Could you check a few things on this model? Use its own coordinates, in mm. A direction names the side the tool comes from. Round coordinates to 2 decimals unless told otherwise and drop trailing zeros. Write each loop counter-clockwise with the first axis right and the second up, starting at its lowest first coordinate (ties: lowest second). Pieces come first, ordered by that corner, then holes. Notation, with made-up numbers: M -19.75,35.5 L 11.25,35.5 A13 cw 11.25,53.5 Z; hole C 20.25,-31 d5. An arc over 180 degrees is marked long. One line per question, with ' | ' between items. Start each with the question number.
```python
from build123d import *

# Parameters (mm, degrees)
SKETCH1_W           = 14.1
SKETCH1_H           = 14.1
BOSS_EXTRUDE1_DEPTH = 250.825
SKETCH2_W           = 10.1
SKETCH2_H           = 10.1
CUT_EXTRUDE1_DEPTH  = 255.432185656
SKETCH3_R           = 1.775
SKETCH3_R_2         = 2.358740524
CUT_EXTRUDE2_DEPTH  = 254.524349476
SKETCH4_R           = 1.775
CUT_EXTRUDE3_DEPTH  = 2
SKETCH5_R           = 1.775
CUT_EXTRUDE4_DEPTH  = 253.531071247


with BuildPart() as part:
    # Sketch1 → Boss-Extrude1 (new body)
    with BuildSketch(Plane.XY):
        with Locations((27.046996237, 18.639517713)):
            Rectangle(SKETCH1_W, SKETCH1_H)
    extrude(amount=BOSS_EXTRUDE1_DEPTH)

    # Sketch2 → Cut-Extrude1 (cut, through all)
    with BuildSketch(Plane.XY.offset(250.825)):
        with Locations((27.046996237, 18.639517713)):
            Rectangle(SKETCH2_W, SKETCH2_H)
    extrude(amount=-CUT_EXTRUDE1_DEPTH, mode=Mode.SUBTRACT)

    # Sketch3 → Cut-Extrude2 (cut, through all)
    with BuildSketch(Plane.XZ.offset(-11.589517713)):
        with Locations(Location((27.046996237, 237.825, 0), (0, 0, 270))):
            Circle(SKETCH3_R)
        with Locations(Location((27.046996237, 208.025, 0), (0, 0, 270))):
            Circle(SKETCH3_R)
        with Locations(Location((27.046996237, 8, 0), (0, 0, 270))):
            Circle(SKETCH3_R_2)
        with Locations(Location((27.046996237, 33, 0), (0, 0, 270))):
            Circle(SKETCH3_R_2)
    extrude(amount=-CUT_EXTRUDE2_DEPTH, mode=Mode.SUBTRACT)

    # Sketch4 → Cut-Extrude3 (cut)
    with BuildSketch(Plane.XZ.offset(-11.589517713)):
        with Locations(Location((27.046996237, 246.825, 0), (0, 0, 270))):
            Circle(SKETCH4_R)
    extrude(amount=-CUT_EXTRUDE3_DEPTH, mode=Mode.SUBTRACT)

    # Sketch5 → Cut-Extrude4 (cut, through all)
    with BuildSketch(Plane(origin=(34.096996237, 0, 0), x_dir=(0, 0, -1), z_dir=(1, 0, 0))):
        with Locations((-193.825, 18.639517713)):
            Circle(SKETCH5_R)
    extrude(amount=-CUT_EXTRUDE4_DEPTH, mode=Mode.SUBTRACT)


solid = part.part
```
1. Which directions (+Z, -Z, +X, -X, +Y, -Y) give clear straight access to the entire face, cutting with the end or side of a thin tool? Please do faces 1 (the face through (27, 25, 250.825)), 2 (the face through (27, 13.59, 127)).
2. If we mould it in two halves opening along Y, with no side actions, what happens to faces 3 (the face through (27, 11.59, 124)), 4 (the face through (27, 23.69, 127)), 5 (the face through (34.097, 19, 124))? For each: released by +Y, released by -Y, zero draft, split by the parting line, or undercut.
3. I need wall thicknesses on line 1 along X through (y, z) = (14, 139.5); line 2 along Y through (x, z) = (25.75, 39); line 3 along X through (y, z) = (13.1, 8). Which ranges of each line are inside material? Lowest first, please. Write a range as from..to.
4. Suppose I cut it at A-A (z = 8). Write out the boundary of the cut face in (x, y).
5. Suppose I cut it at B-B (z = 131). Write out the boundary of the cut face in (x, y), and give its area (3 significant figures).
6. I'm going to push flat-ended pins straight in: P1, Ø2, axis at x = 27.5, y = 14.5, coming from the -Z side; P2, Ø4, axis at x = 25.5, y = 20, coming from the +Z side. Where does each tip first touch, or does it pass through?
Computed:
1) face 1: +Z, +X, -X, +Y, -Y | face 2: +Z, -Z
2) face 3: released by -Y | face 4: undercut | face 5: zero draft
3) line 1: x = 20..22, 32.1..34.1 | line 2: y = 11.59..13.59, 23.69..25.69 | line 3: x = 20..24.69, 29.41..34.1
4) outline: M 20,11.59 L 24.69,11.59 L 24.69,13.59 L 22,13.59 L 22,23.69 L 24.69,23.69 L 24.69,25.69 L 20,25.69 Z; M 29.41,11.59 L 34.1,11.59 L 34.1,25.69 L 29.41,25.69 L 29.41,23.69 L 32.1,23.69 L 32.1,13.59 L 29.41,13.59 Z
5) outline: M 20,11.59 L 34.1,11.59 L 34.1,25.69 L 20,25.69 Z; hole M 22,13.59 L 32.1,13.59 L 32.1,23.69 L 22,23.69 Z | area: 96.8 mm²
6) P1: stops at z = 0 | P2: passes through
